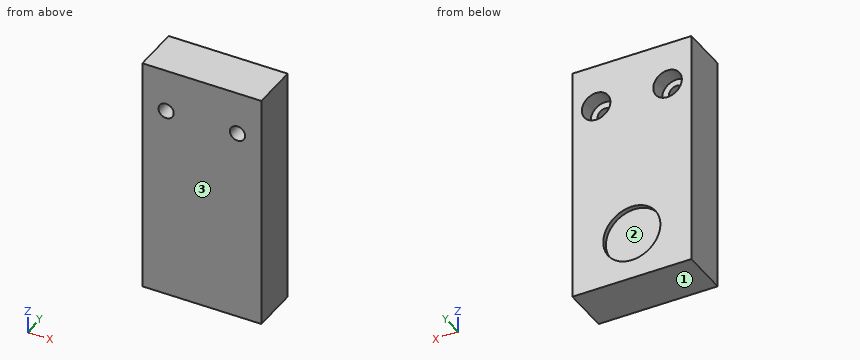
```python
from build123d import *

# Parameters (mm, degrees)
SKETCH_1_W                = 25
SKETCH_1_H                = 50
EXTRUDE_1_DEPTH           = 10
HOLE_WIZARD_1_D           = 3.2
HOLE_WIZARD_1_CBORE_D     = 6
HOLE_WIZARD_1_CBORE_DEPTH = 3.4
SKETCH_5_R                = 6
CUT_EXTRUDE_1_DEPTH       = 1


with BuildPart() as part:
    # 草图1 → 凸台-拉伸1 (new body)
    with BuildSketch(Plane(origin=(0, 0, 0), x_dir=(1, 0, 0), z_dir=(0, 1, 0))):
        Rectangle(SKETCH_1_W, SKETCH_1_H)
    extrude(amount=EXTRUDE_1_DEPTH)

    # 打孔尺寸(%根据)内六角圆柱头螺钉的类型1 (through all)
    with Locations(Plane(origin=(0, 10, 0), x_dir=(1, 0, 0), z_dir=(0, 1, 0))):
        with Locations((-7.5, -16), (7.5, -16)):
            CounterBoreHole(HOLE_WIZARD_1_D / 2, HOLE_WIZARD_1_CBORE_D / 2, HOLE_WIZARD_1_CBORE_DEPTH)

    # 草图5 → 切除-拉伸1 (cut)
    with BuildSketch(Plane(origin=(0, 10, 0), x_dir=(1, 0, 0), z_dir=(0, 1, 0))):
        with Locations((0, 15)):
            Circle(SKETCH_5_R)
    extrude(amount=-CUT_EXTRUDE_1_DEPTH, mode=Mode.SUBTRACT)


solid = part.part
```
Here's how the part is built. I have some questions about the finished solid (model axes, mm). Face numbers are marked on the shaded views. Coordinates: 2 decimals unless noted, no trailing zeros. Order: outer loops, then holes, each group sorted by start corner. A loop starts at its lowest first (then second) coordinate and runs counter-clockwise, first axis right, second up.
1) Will these pins go through, and if not, where does the flat tip stop? pin 1 (11 mm diameter, centred on x = 0, z = -15, fed in from -Y); pin 2 (1.8 mm diameter, centred on x = 8.5, z = 15.5, fed in from +Y).
2) We'd pull the mould along Z, two halves only. Please class the marked faces 1, 2 and 3: +Z half, -Z half, draft (parallel to the pull), parting line (faces both ways), or undercut.
3) Imagine slicing it at D-D on x = 0. List the corners of the cut face in (y, z) for me, and give its area (3 significant figures).
4) I need wall thicknesses on line 1 (X direction, y = 1.5, z = 16); line 2 (X direction, y = 8.6, z = 16); line 3 (Z direction, x = 7.5, y = 5.25). Which ranges of each line are inside material? Lowest first, please.
5) Imagine slicing it at A-A on z = 16. List the corners of the cut face in (x, y) for me.
6) Imagine slicing it at C-C on y = 8. List the corners of the cut face in (x, z) for me, and give its area (3 significant figures).
7) Imagine slicing it at B-B on x = -7.5. List the corners of the cut face in (y, z) for me, and give its area (3 significant figures).
Response values:
1. pin 1: stops at y = 0
1. pin 2: stops at y = 6.6
2. face 1: -Z half
2. face 2: undercut
2. face 3: draft
3. outline: (0, -25) - (10, -25) - (10, -21) - (9, -21) - (9, -9) - (10, -9) - (10, 25) - (0, 25) - close
3. area: 488 mm2
4. line 1: x = -12.5 to -9.1, -5.9 to 5.9, 9.1 to 12.5
4. line 2: x = -12.5 to -10.5, -4.5 to 4.5, 10.5 to 12.5
4. line 3: z = -25 to 14.4, 17.6 to 25
5. outline: (-12.5, 0) - (-9.1, 0) - (-9.1, 6.6) - (-10.5, 6.6) - (-10.5, 10) - (-12.5, 10) - close; (-5.9, 0) - (5.9, 0) - (5.9, 6.6) - (4.5, 6.6) - (4.5, 10) - (-4.5, 10) - (-4.5, 6.6) - (-5.9, 6.6) - close; (9.1, 0) - (12.5, 0) - (12.5, 10) - (10.5, 10) - (10.5, 6.6) - (9.1, 6.6) - close
6. outline: (-12.5, -25) - (12.5, -25) - (12.5, 25) - (-12.5, 25) - close; hole circle Ø6 at (-7.5, 16); hole circle Ø6 at (7.5, 16)
6. area: 1,190 mm2
7. outline: (0, -25) - (10, -25) - (10, 13) - (6.6, 13) - (6.6, 14.4) - (0, 14.4) - close; (0, 17.6) - (6.6, 17.6) - (6.6, 19) - (10, 19) - (10, 25) - (0, 25) - close
7. area: 458 mm2
